```python
from build123d import *

# Parameters (mm, degrees)
F1_DEPTH  = 63.5
F0_W      = 26.6759653056
F0_H      = 19.05
F0_H_2    = 5.927620608
F2_DEPTH  = 25.4
F2_FACE_W = 50.8
F2_FACE_H = 28.575


with BuildPart() as f1:
    # F0 (on Front) → F1 (new body, symmetric)
    with BuildSketch(Plane.XZ):
        Polygon((-41.275, 9.525), (-41.275, -9.525), (41.275, -9.525), (41.275, 9.525), (22.225, 9.525), align=None)
    extrude(amount=F1_DEPTH, both=True)

    # F0 (on Front) → F2 (join, symmetric)
    with BuildSketch(Plane.XZ):
        Polygon((-41.275, 9.525), (-41.275, -9.525), (41.275, -9.525), (41.275, 9.525), (22.225, 9.525), align=None)
        with BuildLine():
            add(Edge.make_bspline(
                [(-41.275, 9.525), (-41.3433387876, 42.0196428895), (13.0519531667, 62.4538473785), (57.15, 61.9252)],
                knots=[0, 0, 0, 0, 111.5045361635, 111.5045361635, 111.5045361635, 111.5045361635], degree=3))
            Line((-41.275, 9.525), (22.225, 9.525))
            Line((22.225, 9.525), (22.225, 27.0002))
            ThreePointArc((22.225, 27.0002), (32.4542956671, 51.6959043329), (57.15, 61.9252))
        make_face()
        with BuildLine():
            Line((22.225, 9.525), (41.275, 9.525))
            Line((41.275, 9.525), (41.275, 27.0002))
            ThreePointArc((41.275, 27.0002), (45.9246798487, 38.2255201513), (57.15, 42.8752))
            Line((57.15, 42.8752), (67.2383028494, 42.8752))
            Line((67.2383028494, 42.8752), (67.2383028494, 61.9252))
            Line((67.2383028494, 61.9252), (57.15, 61.9252))
            ThreePointArc((57.15, 61.9252), (32.4542956671, 51.6959043329), (22.225, 27.0002))
            Line((22.225, 27.0002), (22.225, 9.525))
        make_face()
        with Locations((80.5762855022, 52.4002)):
            Rectangle(F0_W, F0_H)
        with Locations((80.5762855022, 64.889010304)):
            Rectangle(F0_W, F0_H_2)
        Polygon((93.914268155, 42.8752), (67.2383028494, 42.8752), (67.2383028494, 39.277820608), (118.0383028494, 39.277820608), (118.0383028494, 67.852820608), (93.914268155, 67.852820608), (93.914268155, 61.9252), align=None)
    extrude(amount=F2_DEPTH, both=True)

    # F2_face (on face) → F3 (revolve)
    with BuildSketch(Plane(origin=(118.0383028494, 0, 53.565320608), x_dir=(0, 1, 0), z_dir=(1, 0, 0))):
        Rectangle(F2_FACE_W, F2_FACE_H)
    revolve(axis=Axis((118.0383028494, 0, 67.852820608), (0, 1, 0)))


solid = f1.part
```
For this review, take the finished solid that the model builds, in its own axes (mm). A direction names the side the tool comes from. Round coordinates to 2 decimals unless told otherwise and drop trailing zeros. Write each loop counter-clockwise with the first axis right and the second up, starting at its lowest first coordinate (ties: lowest second). Pieces come first, ordered by that corner, then holes. Notation, with made-up numbers: (21, 15) -> (69, 15) arc R28 cw to (69, 42) -> close; hole circle Ø5 at (59.5, 66). An arc over 180 degrees is marked (long way). Use one line per item in the form item = value.
Q1. Consider section B-B (y = 43.5). State the section outline as (x, z) points (3 decimals), then the cut area to 3 significant figures.
Resolved:
outline = (-41.275, -9.525) -> (41.275, -9.525) -> (41.275, 9.525) -> (-41.275, 9.525) -> close
area = 1,570 mm²
Q2. Clearance check with flat-ended pins moving along their axes: pin 1 Ø11 at (x, y) = (79.5, -4) entering from +Z; pin 2 Ø6 at (y, z) = (2.5, 43) entering from -X; pin 3 Ø11 at (y, z) = (-17.5, 10) entering from +X (3 decimals). State where each tip first meets the part, or that it passes through.
Resolved:
pin_1 = 67.85
pin_2 = -22.53
pin_3 = 41.275
Q3. Consider section A-A (z = 2). State the section outline as (x, y) points (3 decimals), then the cut area to 3 significant figures.
Resolved:
outline = (-41.275, -63.5) -> (41.275, -63.5) -> (41.275, 63.5) -> (-41.275, 63.5) -> close
area = 10,500 mm²
Q4. The part is to be moulded in two halves that separate along X. For faces 4 (the flat face through (51, 25.4, 44)), 5 (the cylindrical face through (45.8, -0.4, 38.1)), 6 (the flat face through (-41.275, -1, 0)), say which applies: released by +X, released by -X, zero draft, split by the parting line, or undercut.
Resolved:
face_4 = zero draft
face_5 = undercut
face_6 = released by -X
Q5. Machinability: for faces 1 (the flat face through (1, -45, 9.525)), 2 (the flat face through (1, 44, 9.525)), 3 (the flat face through (67.238, 0, 65)), which of the approach directions +Z, -Z, +X, -X, +Y, -Y give a long, thin tool a straight path to every point of the face, cutting with its end or side? Answer none if there is none.
Resolved:
face_1 = +Z, +X, -X, -Y
face_2 = +Z, +X, -X, +Y
face_3 = +Z, -X, +Y, -Y
Q6. To check wall thickness, follow probe 1 along Y at (x, z) = (87, 48); probe 2 along Z at (x, y) = (-32, 53) (3 decimals); probe 3 along Z at (x, y) = (130.5, 9). State the ranges of each line that lie inside material, in increasing order. Write a range as from..to.
Resolved:
probe_1 = -25.4..25.4
probe_2 = -9.525..9.525
probe_3 = 42.14..93.57
